Could you check a few things on this model? Use its own coordinates, in mm. Round coordinates to 2 decimals unless told otherwise and drop trailing zeros. Write each loop counter-clockwise with the first axis right and the second up, starting at its lowest first coordinate (ties: lowest second). Pieces come first, ordered by that corner, then holes. Notation, with made-up numbers: (69, 44.25) -> (79, 44.25) arc R23 ccw to (79, 70.25) -> close; hole circle Ø10 at (6, 71). An arc over 180 degrees is marked (long way). Answer in a Markdown table with one row per item.
from build123d import *

# Parameters (mm, degrees)
F7_R     = 1.5875
F8_DEPTH = 44.45


# Not quite as in the source:
# - a length typed as a fraction of an inch, garbled in the dataset ("3 / 203.2 mm" for 3/8 in), is restored
# - a feature names something its author has since deleted; it is built from what else it names


with BuildPart() as f5:
    # F4 (on Front) → F5 (revolve)
    with BuildSketch(Plane.XZ):
        with BuildLine():
            ThreePointArc((-57.8191946572, 81.1773013498), (-32.1183318105, 62.7606186977), (-2.5394843148, 51.5892118125))
            Line((-2.5394843148, 51.5892118125), (7.7792656852, 51.5892118125))
            Line((7.7792656852, 51.5892118125), (7.7792656852, 53.1767118125))
            Line((7.7792656852, 53.1767118125), (-2.3548589537, 53.1767118125))
            ThreePointArc((-2.3548589537, 53.1767118125), (-31.4500310941, 64.2035504476), (-56.7346691844, 82.3365945607))
            ThreePointArc((-56.7346691844, 82.3365945607), (-72.7834805037, 92.4895400844), (-91.4394843148, 96.0392118125))
            Line((-91.4394843148, 96.0392118125), (-91.4394843148, 94.4517118125))
            ThreePointArc((-91.4394843148, 94.4517118125), (-73.3664806228, 91.0129673259), (-57.8191946572, 81.1773013498))
        make_face()
        with BuildLine():
            Line((10.1605156852, 53.1767118125), (10.1605156852, 51.5892118125))
            Line((10.1605156852, 51.5892118125), (22.8605156852, 51.5892118125))
            ThreePointArc((22.8605156852, 51.5892118125), (52.439363181, 62.7606186977), (78.1402260277, 81.1773013498))
            ThreePointArc((78.1402260277, 81.1773013498), (93.6875119933, 91.0129673259), (111.7605156852, 94.4517118125))
            Line((111.7605156852, 94.4517118125), (111.7605156852, 96.0392118125))
            ThreePointArc((111.7605156852, 96.0392118125), (93.1045118742, 92.4895400844), (77.0557005549, 82.3365945607))
            ThreePointArc((77.0557005549, 82.3365945607), (51.7710624646, 64.2035504476), (22.6758903242, 53.1767118125))
            Line((22.6758903242, 53.1767118125), (10.3451410463, 53.1767118125))
            Line((10.3451410463, 53.1767118125), (10.1605156852, 53.1767118125))
        make_face()
        Polygon((7.7792656852, 53.1767118125), (7.7792656852, 51.5892118125), (10.1605156852, 51.5892118125), (10.1605156852, 53.1767118125), (9.9758903242, 53.1767118125), align=None)
    revolve(axis=Axis((-40.6394843148, 0, 45.2392118125), (1, 0, 0)))

    # F4 (on Front) → F6 (revolve)
    with BuildSketch(Plane.XZ):
        Polygon((7.7792656852, 94.4517118125), (7.7792656852, 53.1767118125), (9.9758903242, 53.1767118125), (10.1605156852, 53.1767118125), (10.1605156852, 94.4517118125), align=None)
        Polygon((7.7792656852, 53.1767118125), (7.7792656852, 51.5892118125), (10.1605156852, 51.5892118125), (10.1605156852, 53.1767118125), (9.9758903242, 53.1767118125), align=None)
    revolve(axis=Axis((10.1605156852, 0, 73.0204618125), (0, 0, -1)))

    # F7 (on face) → F8 (cut)
    with BuildSketch(Plane.XY.offset(94.4517118125)):
        with Locations((10.1605156852, 0)):
            Circle(F7_R)
    extrude(amount=-F8_DEPTH, mode=Mode.SUBTRACT)


solid = f5.part
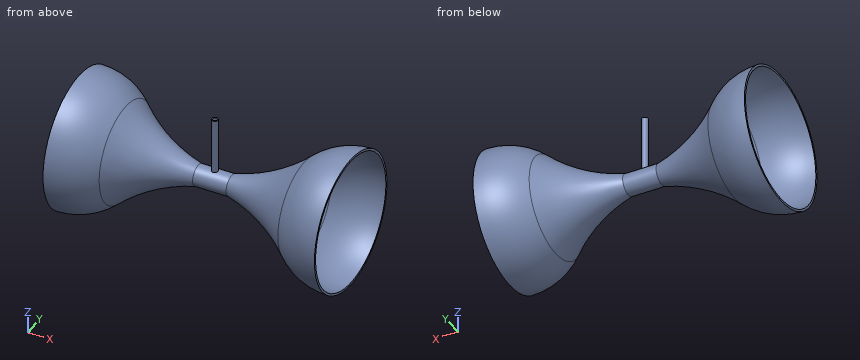
1) Imagine slicing it at D-D, the plane z = 58. Count the separate pieces of the cut face and the enclosed holes in it, plus the area to 3 significant figures.
Findings:
| item | result |
|---|---|
| separate pieces | 3 |
| enclosed holes | 1 |
| area | 694 mm^2 |
2) Please list where these lines run through material, in increasing order: line 1 (X direction, y = 0, z = 66); line 2 (Z direction, x = 12, y = 0); line 3 (Z direction, x = 5.5, y = 0).
Findings:
| item | result |
|---|---|
| line 1 | x = -37.8 to -34.68, 7.78 to 8.57, 11.75 to 12.54, 55 to 58.12 |
| line 2 | z = 37.3 to 38.89, 51.59 to 94.45 |
| line 3 | z = 37.3 to 38.89, 51.59 to 53.18 |
3) For pin 1 (8 mm diameter, centred on x = 82, z = 43.5, fed in from -Y); pin 2 (12 mm diameter, centred on x = 50, y = -18, fed in from +Z); pin 3 (12 mm diameter, centred on x = -40, z = 83.5, fed in from -Y); pin 4 (1 mm diameter, centred on y = 38, z = 64, fed in from -X), each with a flat end and sliding along its axis, tell me the tip position at first contact or that it passes through.
Findings:
| item | result |
|---|---|
| pin 1 | stops at y = -43.75 |
| pin 2 | stops at z = 60.23 |
| pin 3 | passes through |
| pin 4 | stops at x = -67.29 |
4) Imagine slicing it at B-B, the plane z = 4. Please give me the cut outline in (x, y), plus the area to 3 significant figures.
Findings:
| item | result |
|---|---|
| outline | (-91.44, -29.66) arc R29.66 ccw to (-91.44, 29.66) -> (-91.44, 26.86) arc R26.86 cw to (-91.44, -26.86) -> close; (111.76, -29.66) -> (111.76, -26.86) arc R26.86 cw to (111.76, 26.86) -> (111.76, 29.66) arc R29.66 ccw to start |
| area | 499 mm^2 |
5) Imagine slicing it at C-C, the plane x = 68.5. Please give me the cut outline in (y, z).
Findings:
| item | result |
|---|---|
| outline | circle Ø59.63 at (0, 45.24); hole circle Ø55.63 at (0, 45.24) |
6) Imagine slicing it at A-A, the plane y = -40.5. Please give me the cut outline in (x, z) (3 decimals), plus the area to 3 significant figures.
Findings:
| item | result |
|---|---|
| outline | (-91.439, 14.573) arc R30.666 ccw to (-91.439, 75.905) -> (-91.439, 73.197) arc R27.957 cw to (-91.439, 17.282) -> close; (111.761, 14.573) -> (111.761, 17.282) arc R27.957 cw to (111.761, 73.197) -> (111.761, 75.905) arc R30.666 ccw to start |
| area | 499 mm^2 |
